Could you check a few things on this model? Use its own coordinates, in mm. Give positions to 0.01 mm unless a question says otherwise; leave off trailing zeros. Loops run counter-clockwise (first coordinate to the right, second up) from the corner with the lowest first, then second, coordinate; pieces in that order, holes last. Notation, with made-up numbers: M 52,33.5 L 103,33.5 A32 cw 103,63.5 Z; hole C 26,-11.5 d9. An arc over 180 degrees is marked long. Return JSON: item names as keys, results as strings. Group by question number.
1. If we section it at D-D (x = 1.75): Write out the boundary of the cut face in (y, z), plus the area to 3 significant figures.
2. If we section it at B-B (x = 0.25): Write out the boundary of the cut face in (y, z), plus the area to 3 significant figures.
3. If we section it at C-C (z = 11.25): Write out the boundary of the cut face in (x, y).
4. For pin 1 (1.5 mm diameter, centred on x = -2, z = 3.5, fed in from +Y), with a flat end and sliding along its axis, tell me the tip position at first contact or that it passes through.
5. Please list where these lines run through material, in increasing order: line 1 (Y direction, x = 0, z = 0.9); line 2 (Y direction, x = -0.4, z = 2); line 3 (X direction, y = 0.2, z = 9.5).
6. If we section it at A-A (y = 0): Write out the boundary of the cut face in (x, z).
Autodesk Inventor part; units mm, degrees
ref_plane "YZ Plane" through (0, 0, 0) normal (1, 0, 0) x (0, 1, 0)
ref_plane "XZ Plane" through (0, 0, 0) normal (0, 1, 0) x (-1, 0, 0)
ref_plane "XY Plane" through (0, 0, 0) normal (0, 0, 1) x (1, 0, 0)
sketch "スケッチ1" plane through (0, 0, 0) normal (0, 0, 1) x (1, 0, 0)
  circle A0 centre (0, 0) radius 2.257
  dimension "d0" = 4.514
extrude "押し出し1" add sketch "スケッチ1" along normal blind 12.5
sketch "スケッチ2" plane through (0, 0, 12.5) normal (0, 0, 1) x (1, 0, 0)
  circle A0 centre (0, 0) radius 2.257
hole "穴1" at (0, 0, 12.5) direction (0, 0, -1) diameter 2.459 depth 8.8 tip angle 118
sketch "スケッチ3" plane through (0, 0, 0) normal (0, 0, -1) x (-1, 0, 0)
  circle A0 centre (0, 0) radius 2.257
hole "穴2" at (0, 0, 0) direction (0, 0, 1) diameter 2.459 depth 8.8 tip angle 118
properties part number "Shaf"
Answer:
{
 "1": {"outline": "M -1.43,0 L 1.43,0 L 1.43,12.5 L -1.43,12.5 Z", "area": "35.6 mm²"},
 "2": {"outline": "M -2.24,0 L -1.2,0 L -1.2,12.5 L -2.24,12.5 Z; M 1.2,0 L 2.24,0 L 2.24,12.5 L 1.2,12.5 Z", "area": "26.0 mm²"},
 "3": {"outline": "C 0,0 d4.51; hole C 0,0 d2.46"},
 "4": {"pin 1": "stops at y = 1.88"},
 "5": {"line 1": "y = -2.26 to -1.23, 1.23 to 2.26", "line 2": "y = -2.22 to -1.16, 1.16 to 2.22", "line 3": "x = -2.25 to -1.21, 1.21 to 2.25"},
 "6": {"outline": "M -2.26,0 L -1.23,0 L -1.23,12.5 L -2.26,12.5 Z; M 1.23,0 L 2.26,0 L 2.26,12.5 L 1.23,12.5 Z"}
}
